Part model, mm, in its own coordinate system. Coordinates: 2 decimals unless noted, no trailing zeros. Order: outer loops, then holes, each group sorted by start corner. A loop starts at its lowest first (then second) coordinate and runs counter-clockwise, first axis right, second up.
```python
from build123d import *

# Parameters (mm, degrees)
SKETCH_1_W          = 10
SKETCH_1_H          = 10
EXTRUDE_1_DEPTH     = 15
CUT_EXTRUDE_1_DEPTH = 15


with BuildPart() as part:
    # Эскиз1 → Бобышка-Вытянуть1 (new body)
    with BuildSketch(Plane(origin=(0, 0, 0), x_dir=(0, 0, -1), z_dir=(1, 0, 0))):
        with Locations((5, 5)):
            Rectangle(SKETCH_1_W, SKETCH_1_H)
    extrude(amount=EXTRUDE_1_DEPTH)

    # Эскиз2 → Вырез-Вытянуть1 (cut)
    with BuildSketch(Plane(origin=(0, 10, 0), x_dir=(1, 0, 0), z_dir=(0, 1, 0))):
        Polygon((10.050486539, 0), (15, 5.440128208), (15, 0), align=None)
    extrude(amount=-CUT_EXTRUDE_1_DEPTH, mode=Mode.SUBTRACT)


solid = part.part
```
(1) Drop flat-ended pins along their axis: pin 1 (1 mm diameter, centred on y = 8.5, z = -4, fed in from +X); pin 2 (2 mm diameter, centred on x = 4, y = 5.5, fed in from +Z). Give the stop position or say it passes through.
(2) Slice it at C-C, the plane z = -1.5. Give the cut face in (x, y), then the cut area to 3 significant figures.
(3) Slice it at A-A, the plane y = 6. Give the cut face in (x, z).
(4) Slice it at B-B, the plane x = 12. Give the cut face in (y, z).
(5) Probe line 1 (Z direction, x = 12.5, y = 2); line 2 (X direction, y = 2.25, z = -4); line 3 (Z direction, x = 13.5, y = 9). List the from-to ranges inside material, lowest first.
Here are the results:
1. pin 1: stops at x = 14.14
1. pin 2: stops at z = 0
2. outline: (0, 0) - (11.42, 0) - (11.42, 10) - (0, 10) - close
2. area: 114 mm2
3. outline: (0, -10) - (15, -10) - (15, -5.44) - (10.05, 0) - (0, 0) - close
4. outline: (0, -10) - (10, -10) - (10, -2.14) - (0, -2.14) - close
5. line 1: z = -10 to -2.69
5. line 2: x = 0 to 13.69
5. line 3: z = -10 to -3.79
